from build123d import *

# Parameters (mm, degrees)
SKETCH1_W           = 25
SKETCH1_H           = 7
BOSS_EXTRUDE1_DEPTH = 20
SKETCH2_W           = 35
SKETCH2_H           = 17
BOSS_EXTRUDE2_DEPTH = 3
CHAMFER1_SIZE       = 5.196152423
CHAMFER1_SIZE_2     = 3
SKETCH3_W           = 6.2
SKETCH3_H           = 14
CUT_EXTRUDE1_DEPTH  = 7
CUT_EXTRUDE2_REACH  = 40
SKETCH4_R           = 1.65


with BuildPart() as part:
    # Sketch1 → Boss-Extrude1 (new body)
    with BuildSketch(Plane(origin=(0, 0, 0), x_dir=(1, 0, 0), z_dir=(0, 1, 0))):
        with Locations((12.5, 3.5)):
            Rectangle(SKETCH1_W, SKETCH1_H)
    extrude(amount=BOSS_EXTRUDE1_DEPTH)

    # Sketch2 → Boss-Extrude2 (add)
    with BuildSketch(Plane.XZ):
        with Locations((12.5, -3.5)):
            Rectangle(SKETCH2_W, SKETCH2_H)
    extrude(amount=-BOSS_EXTRUDE2_DEPTH)

    # Chamfer1
    # the kernel refuses this chamfer: 5.196152423, 3 mm, written as the material it takes off along each edge
    with BuildSketch(Plane(origin=(30, 0, 18.442891912), x_dir=(-0.9998132206222079, -0.01932676561270063, 0), z_dir=(0, 0, -1)), Plane(origin=(-5, 0, -25.442891912), x_dir=(0.9998132206222079, -0.019326765612700626, 0), z_dir=(0, 0, 1))) as chamfer1_piece_1:
        Polygon((CHAMFER1_SIZE * 0.999813220566, CHAMFER1_SIZE * 0.0193267656116), (-CHAMFER1_SIZE_2 * 0.0193267656127, CHAMFER1_SIZE_2 * 0.999813220622), (0, 0), align=None)
    extrude(amount=43.885783824, mode=Mode.SUBTRACT)
    with BuildSketch(Plane(origin=(-18.442891912, 0, 5), x_dir=(0, -0.019326765612700626, -0.9998132206222079), z_dir=(1, 0, 0)), Plane(origin=(43.442891912, 0, -12), x_dir=(0, -0.019326765612700622, 0.9998132206222079), z_dir=(-1, 0, 0))) as chamfer1_piece_2:
        Polygon((CHAMFER1_SIZE * 0.999813220566, CHAMFER1_SIZE * 0.0193267656116), (-CHAMFER1_SIZE_2 * 0.0193267656127, CHAMFER1_SIZE_2 * 0.999813220622), (0, 0), align=None)
    extrude(amount=61.885783824, mode=Mode.SUBTRACT)

    # Sketch3 → Cut-Extrude1 (cut)
    with BuildSketch(Plane(origin=(0, 0, -7), x_dir=(-1, 0, 0), z_dir=(0, 0, -1))):
        with Locations((-12.5, 13)):
            Rectangle(SKETCH3_W, SKETCH3_H)
    extrude(amount=-CUT_EXTRUDE1_DEPTH, mode=Mode.SUBTRACT)

    # Cut-Extrude2: up to this face of the body (flat: up to its plane)
    cut_extrude2_end = Plane(part.part.faces().sort_by_distance((25, 11.5, -3.5))[0])
    # Sketch4 → Cut-Extrude2 (cut, up to the picked face)
    with BuildSketch(Plane.ZY, mode=Mode.PRIVATE) as cut_extrude2_sk1:
        with Locations((-3.5, 14.5)):
            Circle(SKETCH4_R)
    cut_extrude2_tool1 = split(extrude(cut_extrude2_sk1.sketch, amount=-CUT_EXTRUDE2_REACH, mode=Mode.PRIVATE), bisect_by=cut_extrude2_end, keep=Keep.BOTH, mode=Mode.PRIVATE)
    add(cut_extrude2_tool1.solids().sort_by(Axis((0, 14.5, -3.5), (1, 0, 0)))[0], mode=Mode.SUBTRACT)


solid = part.part
Geometry check sheet. Reference: the model listing, model coordinates, mm. A direction names the side the tool comes from. Give positions to 0.01 mm unless a question says otherwise; leave off trailing zeros. Loops run counter-clockwise (first coordinate to the right, second up) from the corner with the lowest first, then second, coordinate; pieces in that order, holes last.
(1) Section check D-D on y = 14.5. Record the cut outline in (x, z).
From the geometry:
outline: (0, -7) - (9.4, -7) - (9.4, -5.15) - (0, -5.15) - close; (0, -1.85) - (9.4, -1.85) - (9.4, 0) - (0, 0) - close; (15.6, -7) - (25, -7) - (25, -5.15) - (15.6, -5.15) - close; (15.6, -1.85) - (25, -1.85) - (25, 0) - (15.6, 0) - close
(2) Release check for a two-part mould opening along Y. For faces 4 (the flat face through (12.3, 5.7, 0)), 5 (the cylindrical face through (4.634, 15.615, -4.716)), 6 (the flat face through (12.7, 1.5, -9.4)), 7 (the cylindrical face through (20.234, 15.615, -4.716)) record: released by +Y, released by -Y, zero draft, split by the parting line, or undercut.
From the geometry:
face 4: zero draft
face 5: undercut
face 6: released by -Y
face 7: undercut
(3) Section check A-A on y = 10.5. Record the cut outline in (x, z), then the cut area to 3 significant figures.
From the geometry:
outline: (0, -7) - (9.4, -7) - (9.4, 0) - (0, 0) - close; (15.6, -7) - (25, -7) - (25, 0) - (15.6, 0) - close
area: 132 mm2
(4) Section check B-B on z = -3.5. Record the cut outline in (x, y).
From the geometry:
outline: (-5, 3) - (0.2, 0) - (24.8, 0) - (30, 3) - (25, 3) - (25, 12.85) - (15.6, 12.85) - (15.6, 6) - (9.4, 6) - (9.4, 12.85) - (0, 12.85) - (0, 3) - close; (0, 16.15) - (9.4, 16.15) - (9.4, 20) - (0, 20) - close; (15.6, 16.15) - (25, 16.15) - (25, 20) - (15.6, 20) - close
(5) Set-up check for faces 1 (the flat face through (12.3, 5.7, -7)), 2 (the flat face through (13, 6, -4)), 3 (the flat face through (25, 11, -3)): record each of +Z, -Z, +X, -X, +Y, -Y from which the full face is reachable in a straight line by a thin tool's end or side.
From the geometry:
face 1: -Z, +X, -X, +Y
face 2: +Z, -Z, +Y
face 3: +Z, -Z, +X, +Y
(6) Section check C-C on x = 2. Record the cut outline in (y, z).
From the geometry:
outline: (0, -6.8) - (3, -12) - (3, -7) - (20, -7) - (20, 0) - (3, 0) - (3, 5) - (0, -0.2) - close; hole circle Ø3.3 at (14.5, -3.5)
(7) Depth check by flat-ended pin: pin 1 Ø2 at (y, z) = (14.5, -3.5) entering from -X; pin 2 Ø5 at (x, y) = (10, 12) entering from +Z; pin 3 Ø2 at (y, z) = (14, -4) entering from -X; pin 4 Ø2 at (y, z) = (8, -3.5) entering from +X. Enter the tip coordinate at first touch or a pass-through.
From the geometry:
pin 1: passes through
pin 2: stops at z = 0
pin 3: stops at x = 0
pin 4: stops at x = 25
(8) Thickness scan on L1, parallel to Y at x = 20.25, z = -3.5; L2, parallel to X at y = 19.25, z = -6; L3, parallel to Y at x = 1, z = -4.25. Record the ranges inside material, lowest first.
From the geometry:
L1: y = 0 to 12.85, 16.15 to 20
L2: x = 0 to 9.4, 15.6 to 25
L3: y = 0 to 13.03, 15.97 to 20
